```python
from build123d import *

# Parameters (mm, degrees)
SKETCH2_R          = 3.175
CUT_EXTRUDE1_DEPTH = 16.875
CIRPATTERN1_COUNT  = 3
SKETCH3_R          = 15.875
CUT_EXTRUDE2_DEPTH = 54.9750001


with BuildPart() as part:
    # Sketch1 → Revolve1 (revolve)
    with BuildSketch(Plane(origin=(0, 0, 0), x_dir=(1, 0, 0), z_dir=(0, 1, 0))):
        Polygon((-30.1625, -15.875), (-30.1625, -6.35), (-23.8125, -6.35), (-23.8125, -9.525), (23.8125, -9.525), (23.8125, -11.811), (11.1125, -11.811), (11.1125, -15.875), align=None)
    revolve(axis=Axis((-42.066572288, 0, 0), (1, 0, 0)))

    # Sketch2 → Cut-Extrude1 (cut, through all)
    with BuildSketch(Plane(origin=(0, 0, 0), x_dir=(1, 0, 0), z_dir=(0, 1, 0))):
        with Locations((17.4625, 0)):
            Circle(SKETCH2_R)
    cut_extrude1 = extrude(amount=-CUT_EXTRUDE1_DEPTH, mode=Mode.SUBTRACT)

    # CirPattern1: Cut-Extrude1 ×3 about axis
    cirpattern1_axis = Axis((-42.066572288, 0, 0), (1, 0, 0))
    for i in range(1, CIRPATTERN1_COUNT):
        add(cut_extrude1.rotate(cirpattern1_axis, i * 360 / CIRPATTERN1_COUNT), mode=Mode.SUBTRACT)

    # Sketch3 → Cut-Extrude2 (cut, through all)
    with BuildSketch(Plane.ZY.offset(30.1625)):
        Circle(SKETCH3_R)
        Polygon((13.607845243, 1.719070632), (11.811, 0), (13.607845243, -1.719070632), (11.439935716, -2.937276257), (12.75281428, -5.049196365), (10.350058198, -5.689992645), (11.096477095, -8.06206252), (8.609848458, -8.085185868), (8.742907443, -10.568359638), (6.328650275, -9.972357128), (5.839988763, -12.410607852), (3.649799721, -11.232928514), (2.570122111, -13.473051931), (0.741618826, -11.787693689), (-0.861234766, -13.688934607), (-2.213160707, -11.601794718), (-4.238477095, -13.044691178), (-5.028879213, -10.686912317), (-7.34940032, -11.580801826), (-7.528614743, -9.10053191), (-9.998533694, -9.389248105), (-9.555299721, -6.942331615), (-12.019422423, -6.607733394), (-10.981590075, -4.347919092), (-13.285086638, -3.411030492), (-11.717866737, -1.480310822), (-13.716, 0), (-11.717866737, 1.480310822), (-13.285086638, 3.411030492), (-10.981590075, 4.347919092), (-12.019422423, 6.607733394), (-9.555299721, 6.942331615), (-9.998533694, 9.389248105), (-7.528614743, 9.10053191), (-7.34940032, 11.580801826), (-5.028879213, 10.686912317), (-4.238477095, 13.044691178), (-2.213160707, 11.601794718), (-0.861234766, 13.688934607), (0.741618826, 11.787693689), (2.570122111, 13.473051931), (3.649799721, 11.232928514), (5.839988763, 12.410607852), (6.328650275, 9.972357128), (8.742907443, 10.568359638), (8.609848458, 8.085185868), (11.096477095, 8.06206252), (10.350058198, 5.689992645), (12.75281428, 5.049196365), (11.439935716, 2.937276257), align=None, mode=Mode.SUBTRACT)
    extrude(amount=-CUT_EXTRUDE2_DEPTH, mode=Mode.SUBTRACT)


solid = part.part
```
Verification items for the finished model (mm, model axes). A direction names the side the tool comes from. Coordinates: 2 decimals unless noted, no trailing zeros. Loops run counter-clockwise (first coordinate to the right, second up) from the corner with the lowest first, then second, coordinate; pieces in that order, holes last. Notation, with made-up numbers: (33.5, 65) - (92.5, 65) arc R36 ccw to (92.5, 104) - close; hole circle Ø2 at (87.25, -18.75). An arc over 180 degrees is marked (long way). Return JSON: item names as keys, results as strings.
1. Section check B-B, the plane z = 0. Count the separate pieces of the cut face and the enclosed holes in it, then the cut area to 3 significant figures.
Established:
{"separate pieces": "3", "enclosed holes": "0", "area": "343 mm2"}
2. Mould release check, pull along Y, two halves, no side actions. Record for faces 1 (the flat face through (11.112, 12, -4)), 2 (the flat face through (-9.814, 8.149, -9.774)), 3 (the flat face through (-9.814, -12.642, 1.669)): +Y half, -Y half, draft (parallel to the pull), parting line (faces both ways), or undercut.
Established:
{"face 1": "draft", "face 2": "undercut", "face 3": "-Y half"}
3. Tool access check on faces 4 (the flat face through (-9.8, -4, 12.1)), 5 (the flat face through (11.112, 10, 8)), 6 (the flat face through (-9.8, -12.7, -1.5)). Record the directions out of +Z, -Z, +X, -X, +Y, -Y that give a thin tool (end or side, any length) a straight path to the whole face; none if there is none.
Established:
{"face 4": "+Z, +X, -X", "face 5": "+Z, +X, +Y", "face 6": "+X, -X, -Y"}
4. Section check A-A, the plane z = 4.5. Record the boundary of the cut face in (x, y).
Established:
{"outline": "(-30.16, -11.69) - (11.11, -11.69) - (11.11, -10.92) - (23.81, -10.92) - (23.81, -8.39) - (-23.81, -8.39) - (-23.81, -4.48) - (-30.16, -4.48) - close; (-30.16, 4.48) - (-23.81, 4.48) - (-23.81, 8.39) - (23.81, 8.39) - (23.81, 10.92) - (11.11, 10.92) - (11.11, 11.69) - (-30.16, 11.69) - close"}
5. Thickness scan on L1, parallel to Z at x = -20, y = -12; L2, parallel to Y at x = 2, z = 0 (3 decimals); L3, parallel to Y at x = -6, z = 0.5. Record the ranges inside material, lowest first.
Established:
{"L1": "z = -4.59 to -2.77, -1.96 to 0.56, 0.97 to 3.28, 5.08 to 5.92", "L2": "y = -12.667 to -9.525, 9.525 to 12.667", "L3": "y = -12.07 to -9.51, 9.51 to 12.07"}
6. Go/stop test with flat-tipped pins: pin 1 (1.5 mm diameter, centred on x = -21, z = 2.5, fed in from -Y); pin 2 (4 mm diameter, centred on x = -6.5, z = 0, fed in from +Y); pin 3 (4 mm diameter, centred on x = 13.5, y = -4.5, fed in from +Z); pin 4 (7.5 mm diameter, centred on y = 0, z = 0, fed in from -X). Record where each tip stops, or that it passes through.
Established:
{"pin 1": "stops at y = -13.47", "pin 2": "stops at y = 13.69", "pin 3": "stops at z = 11.54", "pin 4": "passes through"}
